Check sheet for the modelled part. Datum: model origin and axes. Units: mm. Round coordinates to 2 decimals unless told otherwise and drop trailing zeros. One line per item, written item: value.
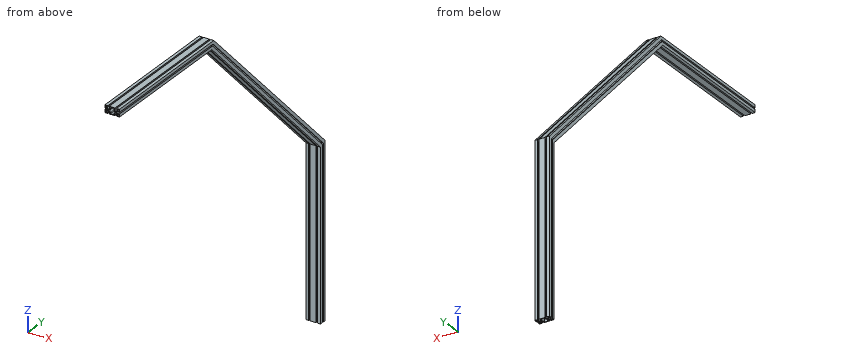
from build123d import *

# Parameters (mm, degrees)
F0_R   = 3
F0_R_2 = 2.5


with BuildPart() as f2:
    # F2: sweep along a path in F1
    with BuildLine(Plane.YZ) as f2_path:
        Line((-15, 0), (-15, 688))
        Line((-15, 688), (-703, 1376))
        Line((-703, 1376), (-1288, 1376))
    # F0 (on Top) → F2 (sweep)
    with BuildSketch(Plane.XY):
        with BuildLine():
            Line((18.15, -15), (30, -15))
            Line((30, -15), (30, -3.15))
            Line((30, -3.15), (27.5, -3.15))
            Line((27.5, -3.15), (27.5, -5.15))
            Line((27.5, -5.15), (21.5477069044, -5.15))
            ThreePointArc((21.5477069044, -5.15), (19.5, 0), (21.5477069044, 5.15))
            Line((21.5477069044, 5.15), (27.5, 5.15))
            Line((27.5, 5.15), (27.5, 3.15))
            Line((27.5, 3.15), (30, 3.15))
            Line((30, 3.15), (30, 15))
            Line((30, 15), (18.15, 15))
            Line((18.15, 15), (18.15, 12.5))
            Line((18.15, 12.5), (20.15, 12.5))
            Line((20.15, 12.5), (20.15, 6.5477069044))
            ThreePointArc((20.15, 6.5477069044), (15, 4.5), (9.85, 6.5477069044))
            Line((9.85, 6.5477069044), (9.85, 12.5))
            Line((9.85, 12.5), (11.85, 12.5))
            Line((11.85, 12.5), (11.85, 15))
            Line((11.85, 15), (-11.85, 15))
            Line((-11.85, 15), (-11.85, 12.5))
            Line((-11.85, 12.5), (-9.85, 12.5))
            Line((-9.85, 12.5), (-9.85, 6.5477069044))
            ThreePointArc((-9.85, 6.5477069044), (-15, 4.5), (-20.15, 6.5477069044))
            Line((-20.15, 6.5477069044), (-20.15, 12.5))
            Line((-20.15, 12.5), (-18.15, 12.5))
            Line((-18.15, 12.5), (-18.15, 15))
            Line((-18.15, 15), (-30, 15))
            Line((-30, 15), (-30, 3.15))
            Line((-30, 3.15), (-27.5, 3.15))
            Line((-27.5, 3.15), (-27.5, 5.15))
            Line((-27.5, 5.15), (-21.5477069044, 5.15))
            ThreePointArc((-21.5477069044, 5.15), (-19.5, 0), (-21.5477069044, -5.15))
            Line((-21.5477069044, -5.15), (-27.5, -5.15))
            Line((-27.5, -5.15), (-27.5, -3.15))
            Line((-27.5, -3.15), (-30, -3.15))
            Line((-30, -3.15), (-30, -15))
            Line((-30, -15), (-18.15, -15))
            Line((-18.15, -15), (-18.15, -12.5))
            Line((-18.15, -12.5), (-20.15, -12.5))
            Line((-20.15, -12.5), (-20.15, -6.5477069044))
            ThreePointArc((-20.15, -6.5477069044), (-15, -4.5), (-9.85, -6.5477069044))
            Line((-9.85, -6.5477069044), (-9.85, -12.5))
            Line((-9.85, -12.5), (-11.85, -12.5))
            Line((-11.85, -12.5), (-11.85, -15))
            Line((-11.85, -15), (11.85, -15))
            Line((11.85, -15), (11.85, -12.5))
            Line((11.85, -12.5), (9.85, -12.5))
            Line((9.85, -12.5), (9.85, -6.5477069044))
            ThreePointArc((9.85, -6.5477069044), (15, -4.5), (20.15, -6.5477069044))
            Line((20.15, -6.5477069044), (20.15, -12.5))
            Line((20.15, -12.5), (18.15, -12.5))
            Line((18.15, -12.5), (18.15, -15))
        make_face()
        with Locations((-25, -10)):
            Circle(F0_R, mode=Mode.SUBTRACT)
        with Locations((25, -10)):
            Circle(F0_R, mode=Mode.SUBTRACT)
        with Locations((-15, 0)):
            Circle(F0_R_2, mode=Mode.SUBTRACT)
        with Locations((-25, 10)):
            Circle(F0_R, mode=Mode.SUBTRACT)
        Polygon((-7, 7), (-7, 12.5), (0, 12.5), (7, 12.5), (7, 7), (10, 0), (7, -7), (7, -12.5), (0, -12.5), (-7, -12.5), (-7, -7), (-10, 0), align=None, mode=Mode.SUBTRACT)
        with Locations((15, 0)):
            Circle(F0_R_2, mode=Mode.SUBTRACT)
        with Locations((25, 10)):
            Circle(F0_R, mode=Mode.SUBTRACT)
    sweep(path=f2_path.line, transition=Transition.RIGHT)


solid = f2.part
Item 1: Material ranges on line 1 along X through (y, z) = (-10, 419); line 2 along Y through (x, z) = (-25, 501), recorded low to high.
Result set:
line 1: -30 to -28, -22 to -20.15, -9.85 to -7, 7 to 9.85, 20.15 to 22, 28 to 30
line 2: -15 to -13, -7 to -5.15, 5.15 to 7, 13 to 15
Item 2: Sectioned sample at A-A (z = 433). State how many separate pieces and enclosed holes the cut face has, then the cut area to 3 significant figures.
Result set:
separate pieces: 1
enclosed holes: 7
area: 706 mm^2
Item 3: Depth check by flat-ended pin: pin 1 (12 mm diameter, centred on x = 23.5, z = 785, fed in from -Y); pin 2 (1.5 mm diameter, centred on x = 7.5, y = -367.5, fed in from +Z); pin 3 (12 mm diameter, centred on x = 21, y = -865.5, fed in from -Z). Enter the tip coordinate at first touch or a pass-through.
Result set:
pin 1: y = -118
pin 2: z = 1083.68
pin 3: z = 1376
